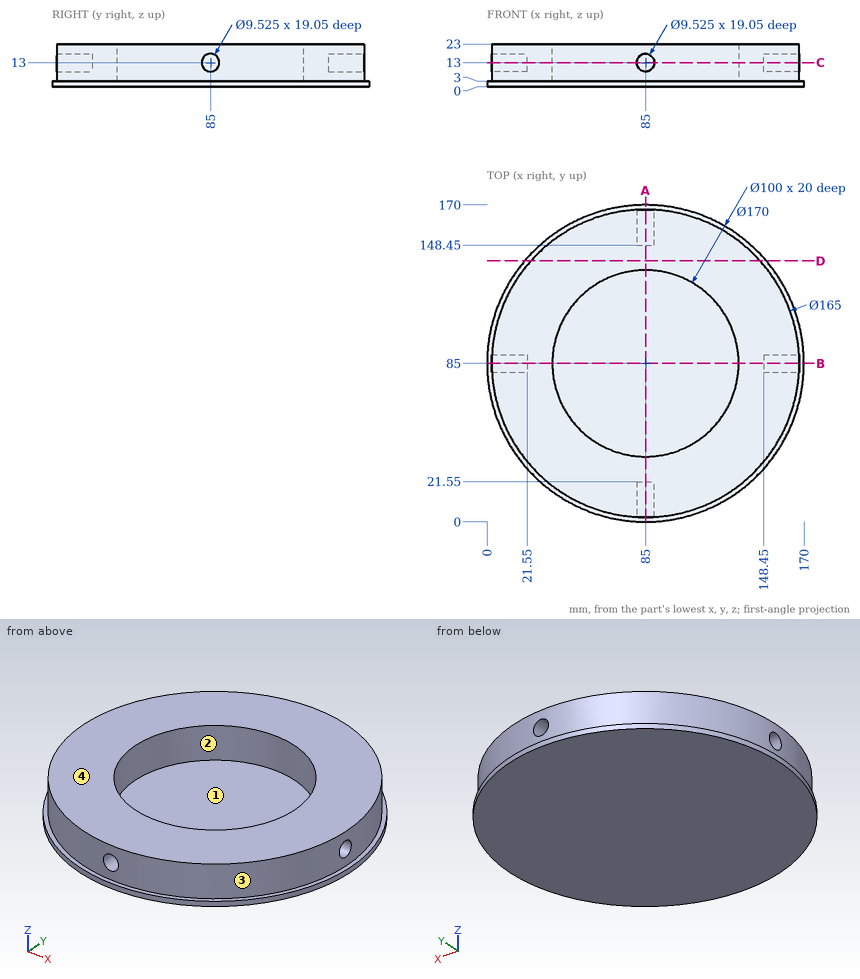
Verification items for this drawing (mm, ordinates from the low corner). Coordinates: 2 decimals unless noted, no trailing zeros. Order: outer loops, then holes, each group sorted by start corner. A loop starts at its lowest first (then second) coordinate and runs counter-clockwise, first axis right, second up. Notation, with made-up numbers: M 42,85 L 57,85 A23 ccw 57,113 Z; hole C 50.25,-31.5 d5. An arc over 180 degrees is marked long. Answer as a JSON object with one key per item and string values.
Q1. Cross-section at D-D on y = 140. Record the cut outline in (x, z).
Results are:
{"outline": "M 20.19,0 L 149.81,0 L 149.81,3 L 146.49,3 L 146.49,23 L 23.51,23 L 23.51,3 L 20.19,3 Z"}
Q2. Scan lines: line 1 (Y direction, x = 85, z = 11.75); line 2 (Y direction, x = 42.5, z = 21.25); line 3 (Z direction, x = 14.5, y = 87). Record each from-to range of solid material in increasing order.
Results are:
{"line 1": "y = 21.55 to 35, 135 to 148.45", "line 2": "y = 14.29 to 58.66, 111.34 to 155.71", "line 3": "z = 0 to 8.68, 17.32 to 23"}
Q3. Cross-section at A-A on x = 85. Record the cut outline in (y, z), and give its area (3 significant figures).
Results are:
{"outline": "M 0,0 L 170,0 L 170,3 L 167.5,3 L 167.5,8.24 L 148.45,8.24 L 148.45,17.76 L 167.5,17.76 L 167.5,23 L 135,23 L 135,3 L 35,3 L 35,23 L 2.5,23 L 2.5,17.76 L 21.55,17.76 L 21.55,8.24 L 2.5,8.24 L 2.5,3 L 0,3 Z", "area": "1,450 mm²"}
Q4. Release check for a two-part mould opening along X. For the marked faces 1, 2, 3 and 4 record: released by +X, released by -X, zero draft, split by the parting line, or undercut.
Results are:
{"face 1": "undercut", "face 2": "undercut", "face 3": "split by the parting line", "face 4": "zero draft"}
Q5. Cross-section at C-C on z = 13. Record the cut outline in (x, y), and give its area (3 significant figures).
Results are:
{"outline": "M 2.64,80.24 A82.5 ccw 80.24,2.64 L 80.24,21.55 L 89.76,21.55 L 89.76,2.64 A82.5 ccw 167.36,80.24 L 148.45,80.24 L 148.45,89.76 L 167.36,89.76 A82.5 ccw 89.76,167.36 L 89.76,148.45 L 80.24,148.45 L 80.24,167.36 A82.5 ccw 2.64,89.76 L 21.55,89.76 L 21.55,80.24 Z; hole C 85,85 d100", "area": "12,800 mm²"}
Q6. Depth check by flat-ended pin: pin 1 Ø8.5 at (y, z) = (85, 13) entering from -X; pin 2 Ø2 at (x, z) = (117, 16.5) entering from -Y; pin 3 Ø3 at (x, z) = (85.5, 15) entering from +Y. Enter the tip coordinate at first touch or a pass-through.
Results are:
{"pin 1": "stops at x = 21.55", "pin 2": "stops at y = 8.55", "pin 3": "stops at y = 148.45"}
